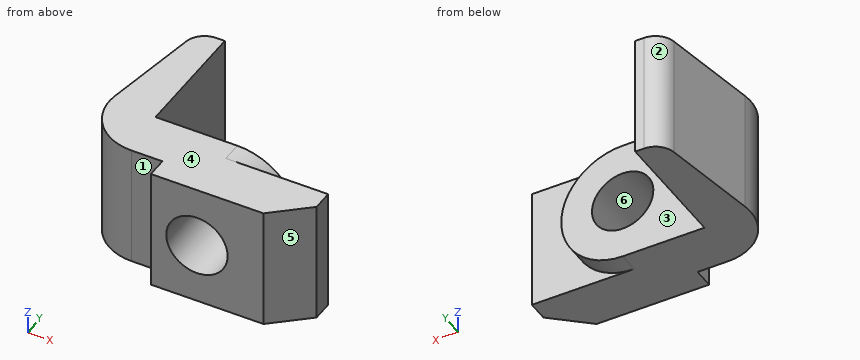
Autodesk Inventor part; units mm, degrees
ref_plane "YZ Plane" through (0, 0, 0) normal (1, 0, 0) x (0, 1, 0)
ref_plane "XZ Plane" through (0, 0, 0) normal (0, 1, 0) x (-1, 0, 0)
ref_plane "XY Plane" through (0, 0, 0) normal (0, 0, 1) x (1, 0, 0)
sketch "Sketch1" plane through (0, 0, 0) normal (0, 0, 1) x (1, 0, 0)
  line L0 (0, 0) -> (19.05, 0)
  line L1 (19.05, 0) -> (19.05, -12.7)
  line L2 (19.05, -12.7) -> (88.9, -12.7)
  line L3 (111.125, 19.05) -> (47.625, 19.05)
  line L4 (47.625, 19.05) -> (47.625, 31.75)
  line L5 (47.625, 31.75) -> (-3.175, 31.75)
  line L6 (-3.175, 31.75) -> (-3.175, 107.95)
  line L7 (-3.175, 107.95) -> (-8.6301, 107.95)
  arc A0 (-8.6301, 107.95) -> (-21.154, 97.3579) centre (-8.6301, 95.25) ccw
  arc A1 (-31.3096, 37.0198) -> (0, 0) centre (0, 31.75) ccw
  line L8 (-31.3096, 37.0198) -> (-21.154, 97.3579)
  line L9 (88.9, -12.7) -> (111.125, 6.35)
  line L10 (111.125, 6.35) -> (111.125, 19.05)
  dimension "d29" = 114.3
  dimension "d30" = 120.65
  dimension "d31" = 19.05
  dimension "d32" = 69.85
  dimension "d33" = 50.8
  dimension "d35" = 31.75
  dimension "d36" = 76.2
  dimension "d37" = 12.7
  dimension "d38" = 31.75
  dimension "d39" = 12.7
  dimension "d40" = 12.7
extrude "Extrusion1" add sketch "Sketch1" along normal mid plane 76.2
sketch "Sketch2" plane through (47.625, 19.05, 38.1) normal (0, 1, 0) x (1, 0, 0)
  line L0 (0, 76.2) -> (0, 0)
  circle A0 centre (0, 38.1) radius 38.1
  point P0 (-47.625, 38.1)
extrude "Extrusion2" add sketch "Sketch2" along normal blind 12.7
hole "Hole1" at (47.625, 31.75, 0) direction (0, -1, 0) diameter 38.1 end through all
properties part number "HW 4 Part 3" material "Iron, Cast"
Geometry: final body of the model. Coordinates: model frame, mm. Face numbers are marked on the shaded views. A direction names the side the tool comes from. Coordinates: 2 decimals unless noted, no trailing zeros. Order: outer loops, then holes, each group sorted by start corner. A loop starts at its lowest first (then second) coordinate and runs counter-clockwise, first axis right, second up. Notation, with made-up numbers: M 50.25,-15.5 L 70.25,-15.5 A24 cw 70.25,22.5 Z; hole C -24,-8 d6. An arc over 180 degrees is marked long. Answer in a Markdown table with one row per item. Add a question column.
Q1. Section query C-C on x = 84. Return the cut outline in (y, z), and give its area (3 significant figures).
Q2. Reachability of the marked faces 1, 2 and 3 from +Z, -Z, +X, -X, +Y, -Y: full face, straight path, thin tool, end or side. Return the list, or none.
Q3. Line query: L1, parallel to Y at x = 13, z = 18; L2, parallel to Y at x = 71.5, z = -8.5; L3, parallel to X at y = 22, z = 0 (3 decimals). Output: solid intervals per line, ascending.
Q4. Section query D-D on y = 17. Return the cut outline in (x, z) (3 decimals), and give its area (3 significant figures).
Q5. Mould query, pull axis X, two halves, no side actions, for the marked faces 4, 5 and 6. Classes: released by +X, released by -X, zero draft, split by the parting line, or undercut.
Q6. Section query B-B on x = 53. Return the cut outline in (y, z), and give its area (3 significant figures).
Q7. Section query A-A on z = 0. Return the cut outline in (x, y) (3 decimals).
Q8. Contact query for flat-ended pins moving along their axis: P1, Ø10, axis at y = 56.5, z = -12.5, coming from the +X side (3 decimals); P2, Ø2, axis at y = 20.5, z = -15, coming from the -X side; P3, Ø3, axis at x = 15.5, z = -17.5, coming from the +Y side. Output: stop coordinate, or through.
Completed:
| question | item | result |
|---|---|---|
| 1 | outline | M -12.7,-38.1 L 19.05,-38.1 L 19.05,-11.33 L 31.75,-11.33 L 31.75,11.33 L 19.05,11.33 L 19.05,38.1 L -12.7,38.1 Z |
| 1 | area | 2,710 mm2 |
| 2 | face 1 | +Z, -Z, -X, -Y |
| 2 | face 2 | +Z, -Z, -X, +Y |
| 2 | face 3 | +Z, -Z, +X, +Y |
| 3 | L1 | y = 0 to 31.75 |
| 3 | L2 | y = -12.7 to 31.75 |
| 3 | L3 | x = -30.216 to 28.575, 66.675 to 85.725 |
| 4 | outline | M -28.116,-38.1 L 111.125,-38.1 L 111.125,38.1 L -28.116,38.1 Z; hole C 47.625,0 d38.1 |
| 4 | area | 9,470 mm2 |
| 5 | face 4 | zero draft |
| 5 | face 5 | released by +X |
| 5 | face 6 | undercut |
| 6 | outline | M -12.7,-38.1 L 19.05,-38.1 L 19.05,-37.72 L 31.75,-37.72 L 31.75,-18.28 L -12.7,-18.28 Z; M -12.7,18.28 L 31.75,18.28 L 31.75,37.72 L 19.05,37.72 L 19.05,38.1 L -12.7,38.1 Z |
| 6 | area | 1,750 mm2 |
| 7 | outline | M -31.31,37.02 A31.75 ccw 0,0 L 19.05,0 L 19.05,-12.7 L 28.575,-12.7 L 28.575,31.75 L -3.175,31.75 L -3.175,107.95 L -8.63,107.95 A12.7 ccw -21.154,97.358 Z; M 66.675,-12.7 L 88.9,-12.7 L 111.125,6.35 L 111.125,19.05 L 85.725,19.05 L 85.725,31.75 L 66.675,31.75 Z |
| 8 | P1 | stops at x = -3.175 |
| 8 | P2 | stops at x = -30.05 |
| 8 | P3 | stops at y = 31.75 |
